Study the drawing (mm; zero at the part's minimum x, y, z) and answer. A direction names the side the tool comes from. Round coordinates to 2 decimals unless told otherwise and drop trailing zeros. Order: outer loops, then holes, each group sorted by start corner. A loop starts at its lowest first (then second) coordinate and runs counter-clockwise, first axis right, second up. Notation, with made-up numbers: (7.25, 24) - (20.25, 24) arc R26 ccw to (20.25, 50) - close; hole circle Ø7 at (-15, -4). An arc over 180 degrees is marked (long way). Put each result on its own line as item: value.
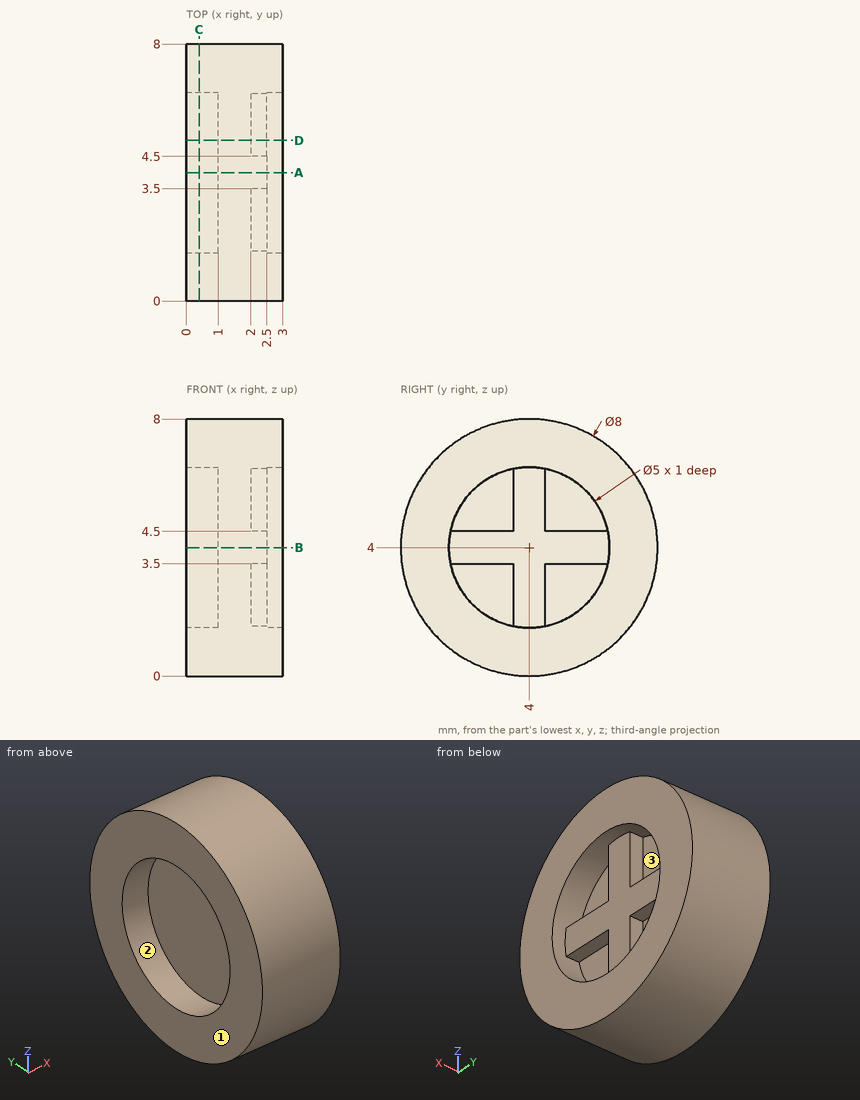
1) Straight lines are drawn through the part: L1, parallel to Y at x = 0.65, z = 4; L2, parallel to X at y = 4, z = 2.75; L3, parallel to X at y = 5.25, z = 3.25. For each, find the intervals that lie inside material, in ascending order. Write a range as from..to.
Findings below:
L1: y = 0..1.5, 6.5..8
L2: x = 1..2.5
L3: x = 1..2
2) A cutting plane is placed at A-A on y = 4. Write down the section's boundary in (x, z), then the cut area to 3 significant figures.
Findings below:
outline: (0, 0) - (3, 0) - (3, 1.5) - (2.5, 1.5) - (2.5, 6.5) - (3, 6.5) - (3, 8) - (0, 8) - (0, 6.5) - (1, 6.5) - (1, 1.5) - (0, 1.5) - close
area: 16.5 mm2
3) A cutting plane is placed at C-C on x = 0.4. Write down the section's boundary in (y, z), then the cut area to 3 significant figures.
Findings below:
outline: circle Ø8 at (4, 4); hole circle Ø5 at (4, 4)
area: 30.6 mm2
4) A cutting plane is placed at D-D on y = 5. Write down the section's boundary in (x, z).
Findings below:
outline: (0, 0.13) - (3, 0.13) - (3, 1.71) - (2, 1.71) - (2, 3.5) - (2.5, 3.5) - (2.5, 4.5) - (2, 4.5) - (2, 6.29) - (3, 6.29) - (3, 7.87) - (0, 7.87) - (0, 6.29) - (1, 6.29) - (1, 1.71) - (0, 1.71) - close
5) Given pin 1 Ø1 at (y, z) = (7, 6.5) entering from -X; pin 2 Ø1.5 at (x, y) = (2.5, 3) entering from +Z; pin 3 Ø0.6 at (x, y) = (2.5, 5.5) entering from -Z; pin 4 Ø0.6 at (x, y) = (2, 2.5) entering from +Z, each flat-ended and moving along its own axis, determine where each tip first touches the part or whether it passes through.
Findings below:
pin 1: stops at x = 0
pin 2: stops at z = 7.99
pin 3: stops at z = 0.18
pin 4: stops at z = 7.82
6) For the marked faces 1, 2 and 3, determine the directions among +Z, -Z, +X, -X, +Y, -Y from which every point of the face is accessible in a straight line to the end or side of a thin tool.
Findings below:
face 1: +Z, -Z, -X, +Y, -Y
face 2: -X
face 3: +X
